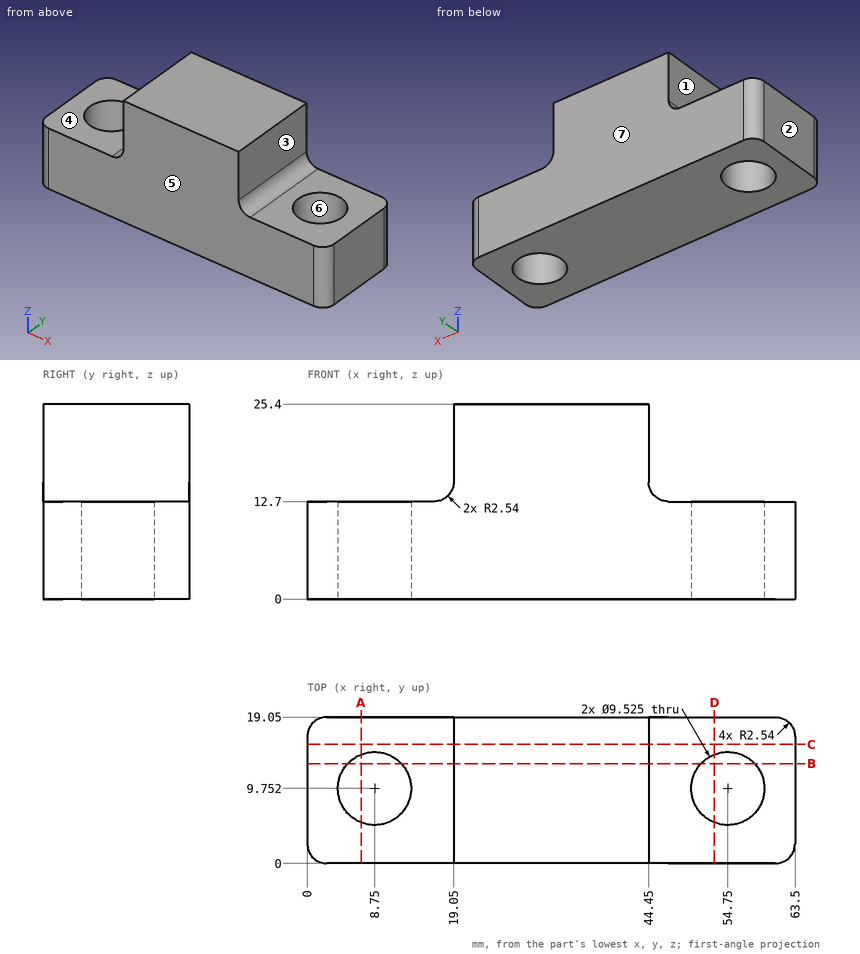
Here's the drawing with two shaded views (mm, measured from the low corner). I have some questions. A direction names the side the tool comes from. Coordinates: 2 decimals unless noted, no trailing zeros. Loops run counter-clockwise (first coordinate to the right, second up) from the corner with the lowest first, then second, coordinate; pieces in that order, holes last. Notation, with made-up numbers: (69.5, 26.5) -> (107.5, 26.5) arc R20 ccw to (107.5, 60.5) -> close; hole circle Ø7 at (61.5, 24). An arc over 180 degrees is marked (long way). Use one line per item in the form item = value. Start each with the question number.
(1) Will these pins go through, and if not, where does the flat tip stop? pin 1 (3 mm diameter, centred on y = 4.5, z = 17.5, fed in from +X); pin 2 (10 mm diameter, centred on x = 52.5, y = 11.5, fed in from +Z); pin 3 (8.5 mm diameter, centred on x = 8.75, y = 9.75, fed in from +Z); pin 4 (11 mm diameter, centred on y = 8, z = 20.5, fed in from -X).
(2) We'd pull the mould along Y, two halves only. Please class the marked faces 4, 5, 6 and 7: pulls with the +Y half, pulls with the -Y half, needs draft (parallel to the pull), parting line crosses it, or undercut.
(3) If we section it at C-C (y = 15.5): Please give me the cut outline in (x, z), then the cut area to 3 significant figures.
(4) If we section it at A-A (x = 7): Please give me the cut outline in (y, z), then the cut area to 3 significant figures.
(5) On a 3-axis mill with a long thin cutter (end or side, diameter ignored), from which of +Z, -Z, +X, -X, +Y, -Y can I reach the whole of each face in a straight line? I mean the marked faces 1, 2 and 3. Say none if no direction works.
(6) Please list where these lines run through material, in increasing order: line 1 along X through (y, z) = (13, 10.5); line 2 along X through (y, z) = (5.75, 2.5); line 3 along Z through (x, y) = (10.5, 15).
(7) If we section it at B-B (y = 13): Please give me the cut outline in (x, z), then the cut area to 3 significant figures.
Verdict:
q1.pin_1 = 44.45
q1.pin_2 = 12.7
q1.pin_3 = through
q1.pin_4 = 19.04
q2.face_4 = needs draft
q2.face_5 = pulls with the -Y half
q2.face_6 = undercut
q2.face_7 = pulls with the +Y half
q3.outline = (0, 0) -> (63.5, 0) -> (63.5, 12.7) -> (46.99, 12.7) arc R2.54 cw to (44.45, 15.24) -> (44.45, 25.4) -> (19.05, 25.4) -> (19.05, 15.24) arc R2.54 cw to (16.51, 12.7) -> (0, 12.7) -> close
q3.area = 1,130 mm²
q4.outline = (0, 0) -> (5.32, 0) -> (5.32, 12.7) -> (0, 12.7) -> close; (14.18, 0) -> (19.05, 0) -> (19.05, 12.7) -> (14.18, 12.7) -> close
q4.area = 129 mm²
q5.face_1 = +Z, -X, +Y, -Y
q5.face_2 = +Z, -Z, -X, +Y, -Y
q5.face_3 = +Z, +X, +Y, -Y
q6.line_1 = 0 to 5.27, 12.23 to 51.27, 58.23 to 63.5
q6.line_2 = 0 to 6.17, 11.33 to 52.17, 57.33 to 63.5
q6.line_3 = 0 to 12.7
q7.outline = (0, 0) -> (5.27, 0) -> (5.27, 12.7) -> (0, 12.7) -> close; (12.23, 0) -> (51.27, 0) -> (51.27, 12.7) -> (46.99, 12.7) arc R2.54 cw to (44.45, 15.24) -> (44.45, 25.4) -> (19.05, 25.4) -> (19.05, 15.24) arc R2.54 cw to (16.51, 12.7) -> (12.23, 12.7) -> close; (58.23, 0) -> (63.5, 0) -> (63.5, 12.7) -> (58.23, 12.7) -> close
q7.area = 955 mm²
